Check sheet for the modelled part. Datum: model origin and axes. Units: mm. Face numbers are marked on the shaded views. A direction names the side the tool comes from. Round coordinates to 2 decimals unless told otherwise and drop trailing zeros. Order: outer loops, then holes, each group sorted by start corner. A loop starts at its lowest first (then second) coordinate and runs counter-clockwise, first axis right, second up.
(1) Mould release check, pull along Y, two halves, no side actions. Record for the marked faces 3, 4, 5 and 6: released by +Y, released by -Y, zero draft, split by the parting line, or undercut.
(2) Tool access check on the marked faces 1 and 2. Record the directions out of +Z, -Z, +X, -X, +Y, -Y that give a thin tool (end or side, any length) a straight path to the whole face; none if there is none.
(3) Thickness scan on probe 1 along Y at (x, z) = (-66.5, 4.5); probe 2 along X at (y, z) = (-46, -8.5); probe 3 along X at (y, z) = (-103, 27.5). Record the ranges inside material, lowest first.
(4) Sectioned sample at D-D, the plane z = 35. Enter the section's corners in (x, y), and give its area (3 significant figures).
(5) Sectioned sample at B-B, the plane z = 20. Enter the section's corners in (x, y).
(6) Depth check by flat-ended pin: pin 1 (13 mm diameter, centred on y = -174, z = -5.5, fed in from +X); pin 2 (0.8 mm diameter, centred on x = -170.5, z = 25, fed in from +Y); pin 3 (22 mm diameter, centred on y = 9.5, z = 18, fed in from -X). Enter the tip coordinate at first touch or a pass-through.
(7) Sectioned sample at A-A, the plane x = -102. Enter the section's corners in (y, z), and give its area (3 significant figures).
(8) Sectioned sample at C-C, the plane y = -42.5. Enter the section's corners in (x, z).
```python
from build123d import *

# Parameters (mm, degrees)
EXTRUDE_1_DEPTH     = 40
SKETCH_2_R          = 20
CUT_EXTRUDE_1_DEPTH = 336
SKETCH_3_W          = 52
SKETCH_3_H          = 244
EXTRUDE_2_DEPTH     = 1.5


with BuildPart() as part:
    # 草图1 → 凸台-拉伸1 (new body)
    with BuildSketch(Plane.XY):
        Polygon((0, 15.741255831), (-169.5, 15.741255831), (-169.5, -268.258744169), (0, -268.258744169), (0, -266.758744169), (-168, -266.758744169), (-168, 14.241255831), (0, 14.241255831), align=None)
    extrude(amount=EXTRUDE_1_DEPTH)

    # 草图2 → 切除-拉伸1 (cut)
    with BuildSketch(Plane(origin=(0, -268.258744169, 0), x_dir=(-1, 0, 0), z_dir=(0, -1, 0))):
        with Locations((0, -20)):
            Circle(SKETCH_2_R)
    extrude(amount=-CUT_EXTRUDE_1_DEPTH, mode=Mode.SUBTRACT)

    # 草图3 → 凸台-拉伸2 (add)
    with BuildSketch(Plane.ZY.offset(169.5)):
        with Locations((14, -126.258744169)):
            Rectangle(SKETCH_3_W, SKETCH_3_H)
    extrude(amount=EXTRUDE_2_DEPTH)


solid = part.part
```
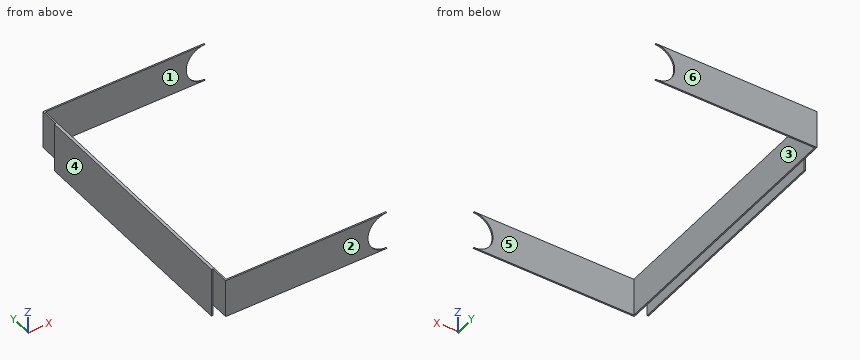
Derived:
1. face 3: undercut
1. face 4: zero draft
1. face 5: undercut
1. face 6: released by +Y
2. face 1: +Z, -Z, +X
2. face 2: +Z, -Z, +X, -X, -Y
3. probe 1: y = -268.26 to -266.76, 14.24 to 15.74
3. probe 2: x = -171 to -169.5
3. probe 3: x = -171 to -168
4. outline: (-171, -248.26) - (-169.5, -248.26) - (-169.5, -268.26) - (-13.23, -268.26) - (-13.23, -266.76) - (-168, -266.76) - (-168, 14.24) - (-13.23, 14.24) - (-13.23, 15.74) - (-169.5, 15.74) - (-169.5, -4.26) - (-171, -4.26) - close
4. area: 1,260 mm2
5. outline: (-171, -248.26) - (-169.5, -248.26) - (-169.5, -268.26) - (-20, -268.26) - (-20, -266.76) - (-168, -266.76) - (-168, 14.24) - (-20, 14.24) - (-20, 15.74) - (-169.5, 15.74) - (-169.5, -4.26) - (-171, -4.26) - close
6. pin 1: stops at x = -168
6. pin 2: stops at y = -4.26
6. pin 3: stops at x = -169.5
7. outline: (-268.26, 0) - (-266.76, 0) - (-266.76, 40) - (-268.26, 40) - close; (14.24, 0) - (15.74, 0) - (15.74, 40) - (14.24, 40) - close
7. area: 120 mm2
8. outline: (-171, -12) - (-169.5, -12) - (-169.5, 0) - (-168, 0) - (-168, 40) - (-171, 40) - close
